Read the model definition and answer for the solid it produces. Units are mm, in the model's axes. A direction names the side the tool comes from. Give positions to 0.01 mm unless a question says otherwise; leave off trailing zeros. Order: outer loops, then holes, each group sorted by start corner. A loop starts at its lowest first (then second) coordinate and runs counter-clockwise, first axis right, second up. Notation, with made-up numbers: M -2,32 L 22,32 A18 cw 22,51 Z; hole C 37.5,-1 d2. An arc over 180 degrees is marked long. One line per item, written item: value. Start each with the question number.
from build123d import *

# Parameters (mm, degrees)
SKETCH10_W          = 155
SKETCH10_H          = 155
BOSS_EXTRUDE3_DEPTH = 3
SKETCH11_R          = 17.5
SKETCH11_R_2        = 12.59
BOSS_EXTRUDE4_DEPTH = 8.4
SKETCH11_4_R        = 2.3
BOSS_EXTRUDE6_DEPTH = 4
SKETCH12_R          = 2.55
CUT_EXTRUDE1_DEPTH  = 37
SKETCH14_R          = 2.55
CUT_EXTRUDE2_DEPTH  = 75
SKETCH15_R          = 1.5
SKETCH15_R_2        = 3.25
CUT_EXTRUDE3_DEPTH  = 95


with BuildPart() as part:
    # Sketch10 → Boss-Extrude3 (new body)
    with BuildSketch(Plane.XZ):
        with Locations((-75.370825338, 0)):
            Rectangle(SKETCH10_W, SKETCH10_H)
    extrude(amount=BOSS_EXTRUDE3_DEPTH)

    # Sketch11 → Boss-Extrude4 (add)
    with BuildSketch(Plane.XZ.offset(3)):
        with Locations(Location((-75.370825338, 0, 0), (0, 0, 270))):
            Circle(SKETCH11_R)
        with Locations(Location((-75.370825338, 0, 0), (0, 0, 270))):
            Circle(SKETCH11_R_2, mode=Mode.SUBTRACT)
    extrude(amount=BOSS_EXTRUDE4_DEPTH)

    # Sketch11_4 → Boss-Extrude6 (add)
    with BuildSketch(Plane.XZ.offset(3)):
        with Locations(Location((-135.260825338, 59.89, 0), (0, 0, 90))):
            Circle(SKETCH11_4_R)
        with Locations(Location((-15.480825338, 59.89, 0), (0, 0, 270))):
            Circle(SKETCH11_4_R)
        with Locations(Location((-135.260825338, -59.89, 0), (0, 0, 270))):
            Circle(SKETCH11_4_R)
        with Locations(Location((-15.480825338, -59.89, 0), (0, 0, 90))):
            Circle(SKETCH11_4_R)
    extrude(amount=BOSS_EXTRUDE6_DEPTH)

    # Sketch12 → Cut-Extrude1 (cut)
    with BuildSketch(Plane.XY):
        with Locations((-75.370825338, -6.9)):
            Circle(SKETCH12_R)
    extrude(amount=-CUT_EXTRUDE1_DEPTH, mode=Mode.SUBTRACT)

    # Sketch14 → Cut-Extrude2 (cut)
    with BuildSketch(Plane(origin=(0, 0, 0), x_dir=(0, 0, -1), z_dir=(1, 0, 0))):
        with Locations((0, -6.9)):
            Circle(SKETCH14_R)
    extrude(amount=-CUT_EXTRUDE2_DEPTH, mode=Mode.SUBTRACT)

    # Sketch15 → Cut-Extrude3 (cut)
    with BuildSketch(Plane(origin=(0, 0, 0), x_dir=(1, 0, 0), z_dir=(0, 1, 0))):
        with Locations(Location((-102.870825338, 30, 0), (0, 0, 270))):
            Circle(SKETCH15_R)
        with Locations(Location((-47.870825338, 30, 0), (0, 0, 270))):
            Circle(SKETCH15_R)
        with Locations(Location((-47.870825338, -30, 0), (0, 0, 270))):
            Circle(SKETCH15_R)
        with Locations(Location((-102.870825338, -30, 0), (0, 0, 270))):
            Circle(SKETCH15_R)
        with Locations(Location((-75.370825338, 0, 0), (0, 0, 270))):
            Circle(SKETCH15_R_2)
    extrude(amount=-CUT_EXTRUDE3_DEPTH, mode=Mode.SUBTRACT)


solid = part.part
Q1. Find section C-C, the plane x = -84.5. Give the vertices of the cut face in (y, z).
Q2. Find section D-D, the plane x = -140. Give the vertices of the cut face in (y, z), then the cut area to 3 significant figures.
Q3. Each of these flat-tipped pins is pushed along its axis until it touches: pin 1 (3.5 mm diameter, centred on x = -102.87, z = 30, fed in from -Y); pin 2 (6 mm diameter, centred on x = -75.37, z = 0, fed in from -Y); pin 3 (1.5 mm diameter, centred on x = -13.5, z = 40, fed in from +Y); pin 4 (4.5 mm diameter, centred on x = -75.37, y = -6.9, fed in from -Z). Where does it stop, or does it pass through?
Q4. Find section B-B, the plane z = -59.89. Give the vertices of the cut face in (x, y), then the cut area to 3 significant figures.
Q5. Find section A-A, the plane z = 0. Give the vertices of the cut face in (x, y), then the cut area to 3 significant figures.
Q6. A tool of negligible diameter and unlimited length cuts with its end or side. For faces 1 (the cylindrical face through (-137.2, -4.97, 61.13)), 2 (the cylindrical face through (-75.92, -9.39, -14.88)), 3 (the flat face through (-15, -7, 60)), from which of +Z, -Z, +X, -X, +Y, -Y can it reach the whole face along a straight path? Write none if from no direction.
Q7. Determine the mould class of faces 4 (the cylindrical face through (-60.42, -9.16, -1.18)), 5 (the flat face through (-16, -7, -60)), 6 (the flat face through (-59, 0, 1)) for opening direction Y: released by +Y, released by -Y, zero draft, split by the parting line, or undercut.
Q8. Consider probe 1 along Y at (x, z) = (-60, 0); probe 2 along X at (y, z) = (-1.9, -30); probe 3 along X at (y, z) = (-0.65, 0). Determine where each line is inside the solid, lowest interval first.
Evaluation:
1. outline: M -11.4,-14.93 L -3,-14.93 L -3,-77.5 L 0,-77.5 L 0,77.5 L -3,77.5 L -3,14.93 L -11.4,14.93 L -11.4,8.67 L -3,8.67 L -3,-8.67 L -11.4,-8.67 Z
2. outline: M -3,-77.5 L 0,-77.5 L 0,77.5 L -3,77.5 Z
2. area: 465 mm2
3. pin 1: y = -3
3. pin 2: through
3. pin 3: y = 0
3. pin 4: z = 12.39
4. outline: M -152.87,-3 L -137.56,-3 L -137.56,-7 L -132.96,-7 L -132.96,-3 L -17.78,-3 L -17.78,-7 L -13.18,-7 L -13.18,-3 L 2.13,-3 L 2.13,0 L -152.87,0 Z
4. area: 502 mm2
5. outline: M -152.87,-3 L -92.87,-3 L -92.87,-11.4 L -87.96,-11.4 L -87.96,-3 L -78.62,-3 L -78.62,0 L -152.87,0 Z; M -72.12,-3 L -62.78,-3 L -62.78,-4.35 L -57.87,-4.35 L -57.87,-3 L 2.13,-3 L 2.13,0 L -72.12,0 Z; M -62.78,-11.4 L -57.87,-11.4 L -57.87,-9.45 L -62.78,-9.45 Z
5. area: 503 mm2
6. face 1: -Y
6. face 2: -Z
6. face 3: +Z, -Z, +X, -X, -Y
7. face 4: undercut
7. face 5: released by -Y
7. face 6: released by +Y
8. probe 1: -11.4 to -9.45, -4.35 to 0
8. probe 2: -152.87 to -104.37, -101.37 to -49.37, -46.37 to 2.13
8. probe 3: -152.87 to -78.62, -72.12 to 2.13
